from build123d import *

# Parameters (mm, degrees)
F1_DEPTH = 6.35
F3_D     = 3.7973
F5_D     = 3.2639


with BuildPart() as f1:
    # F0 (on Right) → F1 (new body)
    with BuildSketch(Plane.YZ):
        with BuildLine():
            Line((0, 9.525), (0, 0))
            Line((0, 0), (152.4, 0))
            Line((152.4, 0), (152.4, 9.525))
            ThreePointArc((152.4, 9.525), (151.4700640303, 11.7700640303), (149.225, 12.7))
            Line((149.225, 12.7), (139.7, 12.7))
            Line((139.7, 12.7), (139.7, 60.325))
            ThreePointArc((139.7, 60.325), (138.7700640303, 62.5700640303), (136.525, 63.5))
            Line((136.525, 63.5), (15.875, 63.5))
            ThreePointArc((15.875, 63.5), (13.6299359697, 62.5700640303), (12.7, 60.325))
            Line((12.7, 60.325), (12.7, 12.7))
            Line((12.7, 12.7), (3.175, 12.7))
            ThreePointArc((3.175, 12.7), (0.9299359697, 11.7700640303), (0, 9.525))
        make_face()
    extrude(amount=F1_DEPTH)

    # F3 (through all)
    with Locations(Plane.YZ.offset(6.35)):
        with Locations((76.2, 57.15), (76.2, 6.35)):
            Hole(F3_D / 2)

    # F5 (through all)
    with Locations(Plane.XY.offset(12.7)):
        with Locations((3.175, 6.35), (3.175, 146.05)):
            Hole(F5_D / 2)


solid = f1.part
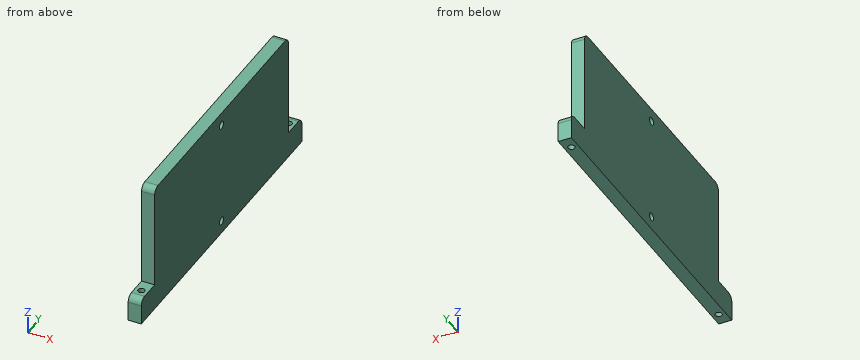
Design review of the part built by this model. Coordinates are the model's own, in mm. Give positions to 0.01 mm unless a question says otherwise; leave off trailing zeros. Loops run counter-clockwise (first coordinate to the right, second up) from the corner with the lowest first, then second, coordinate; pieces in that order, holes last. Notation, with made-up numbers: (59, -35) - (83, -35) arc R14 ccw to (83, -13) - close; hole circle Ø8 at (16, 65.25). An arc over 180 degrees is marked (long way). Use CSV: the item, a comma, the result in double quotes. Start each with the question number.
1. Add section B-B (x = 2.75). State the section outline as (y, z) points (3 decimals), plus the area to 3 significant figures.
2. Insertion check: P1, Ø2.5, axis at y = 76.2, z = 6.35, coming from the -X side. The pin has a flat end and moves straight along its axis. Give the tip position at first contact, or say it passes through.
3. Wall thickness on L1, parallel to Z at x = 5, y = 76.2; L2, parallel to Y at x = 3.75, z = 53.5: over which ranges is each line inside the solid? List them lowest first.
4. Add section C-C (y = 76.2). State the section outline as (x, z) points, plus the area to 3 significant figures.
5. Add section D-D (z = 39). State the section outline as (x, y) points.
6. Add section A-A (y = 6.35). State the section outline as (x, z) points, plus the area to 3 significant figures.
Results found:
1,outline,"(0, 0) - (4.774, 0) - (4.774, 12.7) - (3.175, 12.7) arc R3.175 ccw to (0, 9.525) - close; (7.926, 0) - (144.474, 0) - (144.474, 12.7) - (139.7, 12.7) - (139.7, 60.325) arc R3.175 ccw to (136.525, 63.5) - (15.875, 63.5) arc R3.175 ccw to (12.7, 60.325) - (12.7, 12.7) - (7.926, 12.7) - close; (147.626, 0) - (152.4, 0) - (152.4, 9.525) arc R3.175 ccw to (149.225, 12.7) - (147.626, 12.7) - close; hole circle Ø3.797 at (76.2, 6.35); hole circle Ø3.797 at (76.2, 57.15)"
1,area,"8,280 mm²"
2,P1,"passes through"
3,L1,"z = 0 to 4.45, 8.25 to 55.25, 59.05 to 63.5"
3,L2,"y = 12.7 to 139.7"
4,outline,"(0, 0) - (6.35, 0) - (6.35, 4.45) - (0, 4.45) - close; (0, 8.25) - (6.35, 8.25) - (6.35, 55.25) - (0, 55.25) - close; (0, 59.05) - (6.35, 59.05) - (6.35, 63.5) - (0, 63.5) - close"
4,area,"355 mm²"
5,outline,"(0, 12.7) - (6.35, 12.7) - (6.35, 139.7) - (0, 139.7) - close"
6,outline,"(0, 0) - (1.54, 0) - (1.54, 12.7) - (0, 12.7) - close; (4.81, 0) - (6.35, 0) - (6.35, 12.7) - (4.81, 12.7) - close"
6,area,"39.2 mm²"
